from build123d import *

# Parameters (mm, degrees)
SKETCH1_W           = 12.7
SKETCH1_H           = 12.7
BOSS_EXTRUDE1_DEPTH = 2.54
FILLET1_R           = 0.635
SHELL1_START        = 0.635
SHELL1_OUTLINE_W    = 1.905
SHELL1_OUTLINE_H    = 11.43
SHELL1_DEPTH        = 11.43
SKETCH2_R           = 2.54
BOSS_EXTRUDE2_DEPTH = 1.905


# Read off the part's stored shape, not the designer's step: Shell1
with BuildPart() as part:
    # Sketch1 → Boss-Extrude1 (new body)
    with BuildSketch(Plane(origin=(0, 0, 0), x_dir=(1, 0, 0), z_dir=(0, 1, 0))):
        with Locations((6.35, 6.35)):
            Rectangle(SKETCH1_W, SKETCH1_H)
    extrude(amount=BOSS_EXTRUDE1_DEPTH)

    # Fillet1
    fillet1_edges = [part.edges().sort_by_distance(p)[0] for p in [
        (0, 1.27, -12.7),
        (12.7, 1.27, -12.7),
        (12.7, 1.27, 0),
        (0, 1.27, 0),
    ]]
    fillet(fillet1_edges, radius=FILLET1_R)

    # Shell1 outline → Shell1 (cut)
    with BuildSketch(Plane.YZ.offset(SHELL1_START)):
        with Locations((0.9525, -6.35)):
            Rectangle(SHELL1_OUTLINE_W, SHELL1_OUTLINE_H)
    extrude(amount=SHELL1_DEPTH, mode=Mode.SUBTRACT)

    # Sketch2 → Boss-Extrude2 (add)
    with BuildSketch(Plane(origin=(0, 1.905, 0), x_dir=(-1, 0, 0), z_dir=(0, -1, 0))):
        with Locations(Location((-6.35, 6.35, 0), (0, 0, 270))):
            Circle(SKETCH2_R)
    extrude(amount=BOSS_EXTRUDE2_DEPTH)


solid = part.part
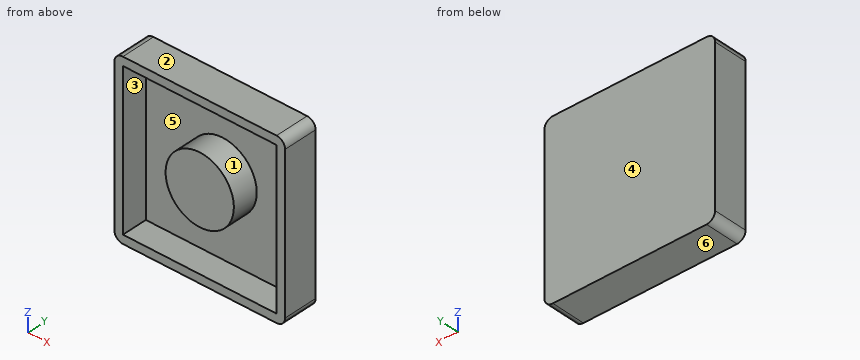
The listing builds one solid part. Answer for the finished solid, in the listing's coordinates (mm). Face numbers are marked on the shaded views. A direction names the side the tool comes from. Round coordinates to 2 decimals unless told otherwise and drop trailing zeros. Order: outer loops, then holes, each group sorted by start corner. A loop starts at its lowest first (then second) coordinate and runs counter-clockwise, first axis right, second up. Notation, with made-up numbers: (-15, -34) -> (16, -34) arc R27 cw to (16, -8) -> close; hole circle Ø6 at (-36, -27). An arc over 180 degrees is marked (long way). Write each question's results on one line, items separated by ' | '. Start each with the question number.
Q1. Which of the six approach directions +Z, -Z, +X, -X, +Y, -Y give full straight-line access (tool end or side, diameter ignored) to the marked faces 1 and 2?
Q2. Find section B-B (z = -6.35). Determine the outline of the cut face in (x, y) (3 decimals).
Q3. Find section C-C (x = 11). Determine the outline of the cut face in (y, z) (3 decimals), then the cut area to 3 significant figures.
Q4. Find section D-D (z = -11). Determine the outline of the cut face in (x, y) (3 decimals), then the cut area to 3 significant figures.
Q5. The mould has two halves that part along Z. Classify the marked faces 3, 4, 5 and 6: pulls with the +Z half, pulls with the -Z half, needs draft (parallel to the pull), parting line crosses it, or undercut.
Q6. Find section A-A (y = 1.7). Determine the outline of the cut face in (x, z) (3 decimals), then the cut area to 3 significant figures.
Q7. Straight lines are drawn through the part: probe 1 along X at (y, z) = (1.6, -2.5) (3 decimals); probe 2 along Z at (x, y) = (7.5, 0.7) (3 decimals); probe 3 along Z at (x, y) = (6.5, 0.6) (3 decimals). For each, find the intervals that lie inside material, in ascending order. Write a range as from..to.
Worked answers:
1) face 1: -Y | face 2: +Z, +X, -X, +Y, -Y
2) outline: (0, 0) -> (0.635, 0) -> (0.635, 1.905) -> (3.81, 1.905) -> (3.81, 0) -> (8.89, 0) -> (8.89, 1.905) -> (12.065, 1.905) -> (12.065, 0) -> (12.7, 0) -> (12.7, 2.54) -> (0, 2.54) -> close
3) outline: (0, -12.7) -> (2.54, -12.7) -> (2.54, 0) -> (0, 0) -> (0, -0.635) -> (1.905, -0.635) -> (1.905, -12.065) -> (0, -12.065) -> close | area: 10.5 mm2
4) outline: (0, 0) -> (0.635, 0) -> (0.635, 1.905) -> (12.065, 1.905) -> (12.065, 0) -> (12.7, 0) -> (12.7, 2.54) -> (0, 2.54) -> close | area: 10.5 mm2
5) face 3: undercut | face 4: needs draft | face 5: undercut | face 6: pulls with the -Z half
6) outline: (0, -12.065) arc R0.635 ccw to (0.635, -12.7) -> (12.065, -12.7) arc R0.635 ccw to (12.7, -12.065) -> (12.7, -0.635) arc R0.635 ccw to (12.065, 0) -> (0.635, 0) arc R0.635 ccw to (0, -0.635) -> close; circle Ø5.08 at (6.35, -6.35); hole (0.635, -12.065) -> (12.065, -12.065) -> (12.065, -0.635) -> (0.635, -0.635) -> close | area: 50.6 mm2
7) probe 1: x = 0..0.635, 12.065..12.7 | probe 2: z = -12.7..-12.065, -8.615..-4.085, -0.635..0 | probe 3: z = -12.7..-12.065, -8.886..-3.814, -0.635..0
